from build123d import *

# Parameters (mm, degrees)
CROQUIS1_W              = 25.4
CROQUIS1_H              = 25.4
SALIENTE_EXTRUIR1_DEPTH = 18
CROQUIS2_W              = 25.4
CROQUIS2_H              = 25.4
CROQUIS2_W_2            = 21.4
CROQUIS2_H_2            = 21.4
CROQUIS2_W_3            = 17.4
CROQUIS2_H_3            = 17.4
CORTAR_EXTRUIR1_DEPTH   = 15
REDONDEO3_R             = 2
REDONDEO4_R             = 1
CROQUIS16_W             = 8
CROQUIS16_H             = 1.5
CORTAR_EXTRUIR13_DEPTH  = 2


with BuildPart() as part:
    # Croquis1 → Saliente-Extruir1 (new body)
    with BuildSketch(Plane.XY):
        Rectangle(CROQUIS1_W, CROQUIS1_H)
    extrude(amount=SALIENTE_EXTRUIR1_DEPTH)

    # Croquis2 → Cortar-Extruir1 (cut)
    # profile 1 of 2: a face of its own
    with BuildSketch(Plane.XY.offset(18)):
        Rectangle(CROQUIS2_W, CROQUIS2_H)
        Rectangle(CROQUIS2_W_2, CROQUIS2_H_2, mode=Mode.SUBTRACT)
    # profile 2 of 2: a face of its own
    with BuildSketch(Plane.XY.offset(18)):
        Rectangle(CROQUIS2_W_3, CROQUIS2_H_3)
    extrude(amount=-CORTAR_EXTRUIR1_DEPTH, mode=Mode.SUBTRACT)

    # Redondeo3
    redondeo3_edges = [part.edges().sort_by_distance(p)[0] for p in [
        (-12.7, 12.7, 1.5),
        (12.7, 12.7, 1.5),
        (12.7, -12.7, 1.5),
        (-12.7, -12.7, 1.5),
        (10.7, 10.7, 10.5),
        (-10.7, 10.7, 10.5),
        (-10.7, -10.7, 10.5),
        (10.7, -10.7, 10.5),
    ]]
    fillet(redondeo3_edges, radius=REDONDEO3_R)

    # Redondeo4
    redondeo4_edges = [part.edges().sort_by_distance(p)[0] for p in [
        (0, 12.7, 0),
        (-12.7, 0, 0),
        (12.7, 0, 0),
        (0, -12.7, 0),
        (12.114213562, -12.114213562, 0),
        (-12.114213562, -12.114213562, 0),
        (-12.114213562, 12.114213562, 0),
        (12.114213562, 12.114213562, 0),
    ]]
    fillet(redondeo4_edges, radius=REDONDEO4_R)

    # Croquis16 → Cortar-Extruir13 (cut)
    with BuildSketch(Plane.XZ.offset(12.7)):
        with Locations((0, 2.25)):
            Rectangle(CROQUIS16_W, CROQUIS16_H)
    extrude(amount=-CORTAR_EXTRUIR13_DEPTH, mode=Mode.SUBTRACT)


solid = part.part
Build history of the part. All positions in model axes, mm. A direction names the side the tool comes from. Round coordinates to 2 decimals unless told otherwise and drop trailing zeros. Write each loop counter-clockwise with the first axis right and the second up, starting at its lowest first coordinate (ties: lowest second). Pieces come first, ordered by that corner, then holes. Notation, with made-up numbers: (50, -35.5) - (103, -35.5) arc R30 ccw to (103, -4.5) - close; hole circle Ø7 at (69, 44). An arc over 180 degrees is marked (long way). Use CSV: the item, a comma, the result in double quotes.
(1) Band-saw the part on D-D (y = -9.5). Write the cut outline in (x, z).
Response:
outline,"(-12.7, 1) arc R1 ccw to (-11.7, 0) - (11.7, 0) arc R1 ccw to (12.7, 1) - (12.7, 3) - (10.53, 3) - (10.53, 18) - (-10.53, 18) - (-10.53, 3) - (-12.7, 3) - close"
(2) Mould opens along X. For faces 1 (the cylindrical face through (-0.15, -12.399, 0.285)), 2 (the flat face through (-10.7, 0, 11)), 3 (the flat face through (0, -12, 1.5)), 4 (the flat face through (-8.7, 0, 11)) say: pulls with the +X half, pulls with the -X half, needs draft (parallel to the pull), parting line crosses it, or undercut.
Response:
face 1,"needs draft"
face 2,"pulls with the -X half"
face 3,"undercut"
face 4,"undercut"
(3) 3-axis set-ups, long thin cutter, end or side, ignore diameter. For faces 5 (the flat face through (4, -12, 2)), 6 (the flat face through (0, 10.7, 11)), 7 (the flat face through (0, -8.7, 11)), 8 (the cylindrical face through (10.13, 10.1, 10.4)): which of +Z, -Z, +X, -X, +Y, -Y reach the whole face in a straight line?
Response:
face 5,"+Z, -Y"
face 6,"+Z, +X, -X, +Y"
face 7,"+Z"
face 8,"+Z, +X, +Y"
(4) Pin check, flat tips, straight feed: P1, Ø1, axis at x = 0, y = -8, coming from the +Z side; P2, Ø2, axis at x = -1.5, y = -11, coming from the +Z side; P3, Ø4, axis at y = -6.5, z = 8, coming from the -X side; P4, Ø8, axis at x = -2, z = 13, coming from the -Y side. Stop position of each tip, or through.
Response:
P1,"z = 3"
P2,"z = 18"
P3,"x = -10.7"
P4,"y = -10.7"
(5) Band-saw the part on A-A (z = 10.75). Write the cut outline in (x, y).
Response:
outline,"(-10.7, -8.7) arc R2 ccw to (-8.7, -10.7) - (8.7, -10.7) arc R2 ccw to (10.7, -8.7) - (10.7, 8.7) arc R2 ccw to (8.7, 10.7) - (-8.7, 10.7) arc R2 ccw to (-10.7, 8.7) - close; hole (-8.7, -8.7) - (8.7, -8.7) - (8.7, 8.7) - (-8.7, 8.7) - close"
(6) Wall check: line 1 (Y direction, x = 2, z = 11.75); line 2 (Z direction, x = 11.75, y = -4.5). Give the ranges that are in metal, low to high.
Response:
line 1,"-10.7 to -8.7, 8.7 to 10.7"
line 2,"0 to 3"
(7) Band-saw the part on B-B (x = 4.5). Write the cut outline in (y, z).
Response:
outline,"(-12.7, 1) arc R1 ccw to (-11.7, 0) - (11.7, 0) arc R1 ccw to (12.7, 1) - (12.7, 3) - (10.7, 3) - (10.7, 18) - (8.7, 18) - (8.7, 3) - (-8.7, 3) - (-8.7, 18) - (-10.7, 18) - (-10.7, 3) - (-12.7, 3) - close"
